Autodesk Inventor part; units mm, degrees
ref_plane "YZ Plane" through (0, 0, 0) normal (1, 0, 0) x (0, 1, 0)
ref_plane "XZ Plane" through (0, 0, 0) normal (0, 1, 0) x (-1, 0, 0)
ref_plane "XY Plane" through (0, 0, 0) normal (0, 0, 1) x (1, 0, 0)
sketch "Block1" plane through (0, 0, 0) normal (0, 0, 1) x (1, 0, 0)
  line L0 (-30.1, 34.1) -> (-9.9, 34.1)
  line L1 (-9.9, 34.1) -> (-9.9, 25.1)
  line L2 (-9.9, 25.1) -> (9.9, 25.1)
  line L3 (9.9, 25.1) -> (9.9, 34.1)
  line L4 (9.9, 34.1) -> (30.1, 34.1)
  line L5 (30.1, 34.1) -> (30.1, 25.1)
  line L6 (30.1, 25.1) -> (50.1, 25.1)
  line L7 (50.1, 25.1) -> (50.1, 16.5667)
  line L8 (50.1, 16.5667) -> (41.1, 16.5667)
  line L9 (41.1, 16.5667) -> (41.1, 6.7667)
  line L10 (41.1, 6.7667) -> (50.1, 6.7667)
  line L11 (50.1, 6.7667) -> (50.1, -6.7667)
  line L12 (50.1, -6.7667) -> (41.1, -6.7667)
  line L13 (41.1, -6.7667) -> (41.1, -16.5667)
  line L14 (41.1, -16.5667) -> (50.1, -16.5667)
  line L15 (50.1, -16.5667) -> (50.1, -25.1)
  line L16 (50.1, -25.1) -> (30.1, -25.1)
  line L17 (30.1, -25.1) -> (30.1, -34.1)
  line L18 (30.1, -34.1) -> (9.9, -34.1)
  line L19 (9.9, -34.1) -> (9.9, -25.1)
  line L20 (9.9, -25.1) -> (-9.9, -25.1)
  line L21 (-9.9, -25.1) -> (-9.9, -34.1)
  line L22 (-9.9, -34.1) -> (-30.1, -34.1)
  line L23 (-30.1, -34.1) -> (-30.1, -25.1)
  line L24 (-30.1, -25.1) -> (-50.1, -25.1)
  line L25 (-50.1, -25.1) -> (-50.1, -16.5667)
  line L26 (-50.1, -16.5667) -> (-41.1, -16.5667)
  line L27 (-41.1, -16.5667) -> (-41.1, -6.7667)
  line L28 (-41.1, -6.7667) -> (-50.1, -6.7667)
  line L29 (-50.1, -6.7667) -> (-50.1, 6.7667)
  line L30 (-50.1, 6.7667) -> (-41.1, 6.7667)
  line L31 (-41.1, 6.7667) -> (-41.1, 16.5667)
  line L32 (-41.1, 16.5667) -> (-50.1, 16.5667)
  line L33 (-50.1, 16.5667) -> (-50.1, 25.1)
  line L34 (-50.1, 25.1) -> (-30.1, 25.1)
  line L35 (-30.1, 25.1) -> (-30.1, 34.1)
  circle A0 centre (-30, 0) radius 4.6
  circle A1 centre (30, 0) radius 4.6
  point P0 (0, 0)
sketch "Block2" plane through (0, 0, 0) normal (0, 0, 1) x (1, 0, 0)
  line L0 (9.8, 34.2) -> (30.2, 34.2)
  line L1 (30.2, 34.2) -> (30.2, 25.2)
  line L2 (30.2, 25.2) -> (50.2, 25.2)
  line L3 (50.2, 25.2) -> (50.2, 16.4667)
  line L4 (50.2, 16.4667) -> (41.2, 16.4667)
  line L5 (41.2, 16.4667) -> (41.2, 6.8667)
  line L6 (41.2, 6.8667) -> (50.2, 6.8667)
  line L7 (50.2, 6.8667) -> (50.2, -6.8667)
  line L8 (50.2, -6.8667) -> (41.2, -6.8667)
  line L9 (41.2, -6.8667) -> (41.2, -16.4667)
  line L10 (41.2, -16.4667) -> (50.2, -16.4667)
  line L11 (50.2, -16.4667) -> (50.2, -25.2)
  line L12 (50.2, -25.2) -> (30.2, -25.2)
  line L13 (30.2, -25.2) -> (30.2, -34.2)
  line L14 (30.2, -34.2) -> (9.8, -34.2)
  line L15 (9.8, -34.2) -> (9.8, -25.2)
  line L16 (9.8, -25.2) -> (-9.8, -25.2)
  line L17 (-9.8, -25.2) -> (-9.8, -34.2)
  line L18 (-9.8, -34.2) -> (-30.2, -34.2)
  line L19 (-30.2, -34.2) -> (-30.2, -25.2)
  line L20 (-30.2, -25.2) -> (-50.2, -25.2)
  line L21 (-50.2, -25.2) -> (-50.2, -16.4667)
  line L22 (-50.2, -16.4667) -> (-41.2, -16.4667)
  line L23 (-41.2, -16.4667) -> (-41.2, -6.8667)
  line L24 (-41.2, -6.8667) -> (-50.2, -6.8667)
  line L25 (-50.2, -6.8667) -> (-50.2, 6.8667)
  line L26 (-50.2, 6.8667) -> (-41.2, 6.8667)
  line L27 (-41.2, 6.8667) -> (-41.2, 16.4667)
  line L28 (-41.2, 16.4667) -> (-50.2, 16.4667)
  line L29 (-50.2, 16.4667) -> (-50.2, 25.2)
  line L30 (-50.2, 25.2) -> (-30.2, 25.2)
  line L31 (-30.2, 25.2) -> (-30.2, 34.2)
  line L32 (-30.2, 34.2) -> (-9.8, 34.2)
  line L33 (-9.8, 34.2) -> (-9.8, 25.2)
  line L34 (-9.8, 25.2) -> (9.8, 25.2)
  line L35 (9.8, 25.2) -> (9.8, 34.2)
  circle A0 centre (30, 0) radius 4.7
  circle A1 centre (-30, 0) radius 4.7
  point P0 (0, 0)
sketch "Block3" plane through (0, 0, 0) normal (0, 0, 1) x (1, 0, 0)
  line L0 (9.9, 34.1) -> (30.1, 34.1)
  line L1 (30.1, 34.1) -> (30.1, 25.1)
  line L2 (30.1, 25.1) -> (50.1, 25.1)
  line L3 (50.1, 25.1) -> (50.1, 16.5667)
  line L4 (50.1, 16.5667) -> (41.1, 16.5667)
  line L5 (41.1, 16.5667) -> (41.1, 6.7667)
  line L6 (41.1, 6.7667) -> (50.1, 6.7667)
  line L7 (50.1, 6.7667) -> (50.1, -6.7667)
  line L8 (50.1, -6.7667) -> (41.1, -6.7667)
  line L9 (41.1, -6.7667) -> (41.1, -16.5667)
  line L10 (41.1, -16.5667) -> (50.1, -16.5667)
  line L11 (50.1, -16.5667) -> (50.1, -25.1)
  line L12 (50.1, -25.1) -> (30.1, -25.1)
  line L13 (30.1, -25.1) -> (30.1, -34.1)
  line L14 (30.1, -34.1) -> (9.9, -34.1)
  line L15 (9.9, -34.1) -> (9.9, -25.1)
  line L16 (9.9, -25.1) -> (-9.9, -25.1)
  line L17 (-9.9, -25.1) -> (-9.9, -34.1)
  line L18 (-9.9, -34.1) -> (-30.1, -34.1)
  line L19 (-30.1, -34.1) -> (-30.1, -25.1)
  line L20 (-30.1, -25.1) -> (-50.1, -25.1)
  line L21 (-50.1, -25.1) -> (-50.1, -16.5667)
  line L22 (-50.1, -16.5667) -> (-41.1, -16.5667)
  line L23 (-41.1, -16.5667) -> (-41.1, -6.7667)
  line L24 (-41.1, -6.7667) -> (-50.1, -6.7667)
  line L25 (-50.1, -6.7667) -> (-50.1, 6.7667)
  line L26 (-50.1, 6.7667) -> (-41.1, 6.7667)
  line L27 (-41.1, 6.7667) -> (-41.1, 16.5667)
  line L28 (-41.1, 16.5667) -> (-50.1, 16.5667)
  line L29 (-50.1, 16.5667) -> (-50.1, 25.1)
  line L30 (-50.1, 25.1) -> (-30.1, 25.1)
  line L31 (-30.1, 25.1) -> (-30.1, 34.1)
  line L32 (-30.1, 34.1) -> (-9.9, 34.1)
  line L33 (-9.9, 34.1) -> (-9.9, 25.1)
  line L34 (-9.9, 25.1) -> (9.9, 25.1)
  line L35 (9.9, 25.1) -> (9.9, 34.1)
  circle A0 centre (-30, 0) radius 4.6
  circle A1 centre (30, 0) radius 4.6
  point P0 (0, 0)
sketch "Block4" plane through (10, 0, 0) normal (0, 1, 0) x (1, 0, 0)
  line L0 (-30.08, 30.58) -> (-9.92, 30.58)
  line L1 (-9.92, 30.58) -> (-9.92, 25.08)
  line L2 (-9.92, 25.08) -> (9.92, 25.08)
  line L3 (9.92, 25.08) -> (9.92, 30.58)
  line L4 (9.92, 30.58) -> (30.08, 30.58)
  line L5 (30.08, 30.58) -> (30.08, 25.08)
  line L6 (30.08, 25.08) -> (50.08, 25.08)
  line L7 (50.08, 25.08) -> (50.08, 16.5867)
  line L8 (50.08, 16.5867) -> (44.58, 16.5867)
  line L9 (44.58, 16.5867) -> (44.58, 6.7467)
  line L10 (44.58, 6.7467) -> (50.08, 6.7467)
  line L11 (50.08, 6.7467) -> (50.08, -6.7467)
  line L12 (50.08, -6.7467) -> (44.58, -6.7467)
  line L13 (44.58, -6.7467) -> (44.58, -16.5867)
  line L14 (44.58, -16.5867) -> (50.08, -16.5867)
  line L15 (50.08, -16.5867) -> (50.08, -25.08)
  line L16 (50.08, -25.08) -> (30.08, -25.08)
  line L17 (30.08, -25.08) -> (30.08, -30.58)
  line L18 (30.08, -30.58) -> (9.92, -30.58)
  line L19 (9.92, -30.58) -> (9.92, -25.08)
  line L20 (9.92, -25.08) -> (-9.92, -25.08)
  line L21 (-9.92, -25.08) -> (-9.92, -30.58)
  line L22 (-9.92, -30.58) -> (-30.08, -30.58)
  line L23 (-30.08, -30.58) -> (-30.08, -25.08)
  line L24 (-30.08, -25.08) -> (-50.08, -25.08)
  line L25 (-50.08, -25.08) -> (-50.08, -16.5867)
  line L26 (-50.08, -16.5867) -> (-44.58, -16.5867)
  line L27 (-44.58, -16.5867) -> (-44.58, -6.7467)
  line L28 (-44.58, -6.7467) -> (-50.08, -6.7467)
  line L29 (-50.08, -6.7467) -> (-50.08, 6.7467)
  line L30 (-50.08, 6.7467) -> (-44.58, 6.7467)
  line L31 (-44.58, 6.7467) -> (-44.58, 16.5867)
  line L32 (-44.58, 16.5867) -> (-50.08, 16.5867)
  line L33 (-50.08, 16.5867) -> (-50.08, 25.08)
  line L34 (-50.08, 25.08) -> (-30.08, 25.08)
  line L35 (-30.08, 25.08) -> (-30.08, 30.58)
  circle A0 centre (-30, 0) radius 4.88
  circle A1 centre (30, 0) radius 4.88
  point P0 (0, 0)
sketch "Block5" plane through (10, 0, 0) normal (0, 1, 0) x (1, 0, 0)
  line L0 (-30.08, 30.58) -> (-9.92, 30.58)
  line L1 (-9.92, 30.58) -> (-9.92, 25.08)
  line L2 (-9.92, 25.08) -> (9.92, 25.08)
  line L3 (9.92, 25.08) -> (9.92, 30.58)
  line L4 (9.92, 30.58) -> (30.08, 30.58)
  line L5 (30.08, 30.58) -> (30.08, 25.08)
  line L6 (30.08, 25.08) -> (50.08, 25.08)
  line L7 (50.08, 25.08) -> (50.08, 16.5867)
  line L8 (50.08, 16.5867) -> (44.58, 16.5867)
  line L9 (44.58, 16.5867) -> (44.58, 6.7467)
  line L10 (44.58, 6.7467) -> (50.08, 6.7467)
  line L11 (50.08, 6.7467) -> (50.08, -6.7467)
  line L12 (50.08, -6.7467) -> (44.58, -6.7467)
  line L13 (44.58, -6.7467) -> (44.58, -16.5867)
  line L14 (44.58, -16.5867) -> (50.08, -16.5867)
  line L15 (50.08, -16.5867) -> (50.08, -25.08)
  line L16 (50.08, -25.08) -> (30.08, -25.08)
  line L17 (30.08, -25.08) -> (30.08, -30.58)
  line L18 (30.08, -30.58) -> (9.92, -30.58)
  line L19 (9.92, -30.58) -> (9.92, -25.08)
  line L20 (9.92, -25.08) -> (-9.92, -25.08)
  line L21 (-9.92, -25.08) -> (-9.92, -30.58)
  line L22 (-9.92, -30.58) -> (-30.08, -30.58)
  line L23 (-30.08, -30.58) -> (-30.08, -25.08)
  line L24 (-30.08, -25.08) -> (-50.08, -25.08)
  line L25 (-50.08, -25.08) -> (-50.08, -16.5867)
  line L26 (-50.08, -16.5867) -> (-44.58, -16.5867)
  line L27 (-44.58, -16.5867) -> (-44.58, -6.7467)
  line L28 (-44.58, -6.7467) -> (-50.08, -6.7467)
  line L29 (-50.08, -6.7467) -> (-50.08, 6.7467)
  line L30 (-50.08, 6.7467) -> (-44.58, 6.7467)
  line L31 (-44.58, 6.7467) -> (-44.58, 16.5867)
  line L32 (-44.58, 16.5867) -> (-50.08, 16.5867)
  line L33 (-50.08, 16.5867) -> (-50.08, 25.08)
  line L34 (-50.08, 25.08) -> (-30.08, 25.08)
  line L35 (-30.08, 25.08) -> (-30.08, 30.58)
  circle A0 centre (-30, 0) radius 4.83
  circle A1 centre (30, 0) radius 4.83
  point P0 (0, 0)
sketch "Sketch10" plane through (0, 0, 0) normal (0, 0, 1) x (1, 0, 0)
  line L0 (50, -25) -> (-50, -25)
  line L1 (-50, -25) -> (-50, 25)
  line L2 (-50, 25) -> (50, 25)
  line L3 (50, 25) -> (50, -25)
  line L4 (50, -25) -> (-50, 25) construction
  line L5 (-50, -25) -> (50, 25) construction
  point P0 (0, 0)
  dimension "d21" = 100
  dimension "d22" = 50
extrude "Extrusion2" add sketch "Sketch10" against normal blind 5.5
sketch "Sketch16" plane through (0, 0, -5.5) normal (0, 0, -1) x (-1, 0, 0)
  line L0 (0, -49.304) -> (0, 48.0007)
  point P0 (0, 0)
  point P1 (-30, 0)
  point P2 (30, 0)
  dimension "d52" = 60
hole "Hole5" at (30, 0, -5.5) at (-30, 0, -5.5) direction (0, 0, 1) diameter 5 end through all
sketch "Sketch35" plane through (0, 0, 0) normal (0, 0, 1) x (1, 0, 0)
  line L0 (-50, 25) -> (50, 25)
  line L1 (-50, -25) -> (-50, 25)
  line L2 (0, -49.304) -> (0, 48.0007)
  line L3 (-213.651, 0) -> (108.296, 0)
  line L4 (50, 25) -> (50, -25)
  line L5 (-30, 25) -> (-30, 30.5)
  line L6 (-30, 30.5) -> (-10, 30.5)
  line L7 (-10, 30.5) -> (-10, 25)
  line L8 (-30, 25) -> (-10, 25)
  line L9 (30, 25) -> (30, 30.5)
  line L10 (30, 30.5) -> (10, 30.5)
  line L11 (10, 30.5) -> (10, 25)
  line L12 (30, 25) -> (10, 25)
  line L13 (-30, -25) -> (-30, -30.5)
  line L14 (-30, -30.5) -> (-10, -30.5)
  line L15 (-10, -30.5) -> (-10, -25)
  line L16 (-30, -25) -> (-10, -25)
  line L17 (30, -25) -> (30, -30.5)
  line L18 (30, -25) -> (10, -25)
  line L19 (30, -30.5) -> (10, -30.5)
  line L20 (10, -30.5) -> (10, -25)
  point P0 (0, 0)
  point P1 (-50, 16.6667)
  point P2 (-50, 4.1667)
  dimension "d129" = 20
  dimension "d130" = 20
  dimension "d131" = 5.5
extrude "Extrusion6" add sketch "Sketch35" against normal blind 5.5 contours L5 L6 L7 L0 | L11 L10 L9 L0 | L16 L15 L14 L13 | L17 L19 L20 L18
sketch "Sketch36" plane through (0, 0, 0) normal (0, 0, 1) x (1, 0, 0)
  line L0 (-50, 25) -> (-30, 25)
  line L1 (-50, -25) -> (-50, 25)
  line L2 (-50, 16.6667) -> (-44.5, 16.6667)
  line L3 (-44.5, 16.6667) -> (-44.5, 6.6667)
  line L4 (-44.5, 6.6667) -> (-50, 6.6667)
  line L5 (-50, 6.6667) -> (-50, 16.6667)
  line L6 (-211.2102, 0) -> (93.6517, 0)
  line L7 (0, -49.304) -> (0, 48.0007)
  line L8 (-50, -16.6667) -> (-44.5, -16.6667)
  line L9 (-44.5, -16.6667) -> (-44.5, -6.6667)
  line L10 (-44.5, -6.6667) -> (-50, -6.6667)
  line L11 (-50, -6.6667) -> (-50, -16.6667)
  line L12 (50, 16.6667) -> (44.5, 16.6667)
  line L13 (44.5, 16.6667) -> (44.5, 6.6667)
  line L14 (44.5, 6.6667) -> (50, 6.6667)
  line L15 (50, 6.6667) -> (50, 16.6667)
  line L16 (44.5, -16.6667) -> (44.5, -6.6667)
  line L17 (44.5, -6.6667) -> (50, -6.6667)
  line L18 (50, -6.6667) -> (50, -16.6667)
  line L19 (50, -16.6667) -> (44.5, -16.6667)
  point P0 (0, 0)
  dimension "d144" = 5.5
  dimension "d145" = 10
  dimension "d146" = 8.3333
extrude "Extrusion7" cut sketch "Sketch36" against normal through all
equation "\"d23\" = Wt"
equation "\"d129\" = 0.2 * d21"
equation "\"d130\" = 0.2 * d21"
equation "\"d131\" = Wt"
equation "\"d142\" = Wt"
equation "\"d144\" = Wt"
equation "\"d145\" = 0.2 * d22"
equation "\"d146\" = 0.166667 * d22"
equation "\"d147\" = Wt"
properties part number "holder_plate" material "Wood (Birch)"
For this review, take the finished solid that the model builds, in its own axes (mm). A direction names the side the tool comes from. Give positions to 0.01 mm unless a question says otherwise; leave off trailing zeros. Write each loop counter-clockwise with the first axis right and the second up, starting at its lowest first coordinate (ties: lowest second). Pieces come first, ordered by that corner, then holes. Notation, with made-up numbers: M 8.25,6 L 24.25,6 A27 ccw 24.25,45 Z; hole C 59,59 d3. An arc over 180 degrees is marked long. Answer as a JSON object with one key per item and string values. Group by question number.
Item 1: Consider section D-D on x = -5.5. Write out the cut boundary in (y, z).
Item 2: For pin 1 Ø4.5 at (x, y) = (30, 0) entering from +Z; pin 2 Ø3 at (y, z) = (-14, -3) entering from -X; pin 3 Ø3 at (y, z) = (28, -4) entering from +X; pin 4 Ø3 at (y, z) = (-27, -3.5) entering from -X, all flat-tipped, find the tip position at first contact; note any pin that passes through.
Item 3: For probe 1 along X at (y, z) = (0, -3); probe 2 along X at (y, z) = (26, -3.5); probe 3 along X at (y, z) = (1, -4.6), list the stretches that pass through material, from the lowest coordinate up. Write a range as [from, to].
Item 4: Consider section B-B on y = 0. Write out the cut boundary in (x, z).
Item 5: Tool access review of faces 1 (the flat face through (10, 28, -3)), 2 (the flat face through (44.5, -12, -3)), 3 (the flat face through (-30, 28, -3)): name each direction out of +Z, -Z, +X, -X, +Y, -Y from which nothing blocks a thin tool from reaching the whole face with its end or side.
Item 6: Consider section C-C on z = -1.4. Count the separate pieces of the cut face and the enclosed holes in it, plus the area to 3 significant figures.
Item 7: Draft analysis for pull direction X (two halves, no side actions). For faces 4 (the flat face through (-44.5, 12, -3)), 5 (the flat face through (-47, 16.667, -3)), 6 (the cylindrical face through (27.52, -0.33, -2.71)), state which applies: +X half, -X half, draft (parallel to the pull), parting line (faces both ways), or undercut.
Item 8: Consider section A-A on y = 26. Write out the cut boundary in (x, z).
Check result:
{
 "1": {"outline": "M -25,-5.5 L 25,-5.5 L 25,0 L -25,0 Z"},
 "2": {"pin 1": "passes through", "pin 2": "stops at x = -44.5", "pin 3": "stops at x = 30", "pin 4": "stops at x = -30"},
 "3": {"probe 1": "x = [-50, -32.5], [-27.5, 27.5], [32.5, 50]", "probe 2": "x = [-30, -10], [10, 30]", "probe 3": "x = [-50, -32.29], [-27.71, 27.71], [32.29, 50]"},
 "4": {"outline": "M -50,-5.5 L -32.5,-5.5 L -32.5,0 L -50,0 Z; M -27.5,-5.5 L 27.5,-5.5 L 27.5,0 L -27.5,0 Z; M 32.5,-5.5 L 50,-5.5 L 50,0 L 32.5,0 Z"},
 "5": {"face 1": "+Z, -Z, +Y", "face 2": "+Z, -Z, +X", "face 3": "+Z, -Z, -X, +Y"},
 "6": {"separate pieces": "1", "enclosed holes": "2", "area": "5,180 mm^2"},
 "7": {"face 4": "-X half", "face 5": "draft", "face 6": "undercut"},
 "8": {"outline": "M -30,-5.5 L -10,-5.5 L -10,0 L -30,0 Z; M 10,-5.5 L 30,-5.5 L 30,0 L 10,0 Z"}
}
